```python
from build123d import *

# Parameters (mm, degrees)
SKETCH2_R           = 88.9
BOSS_EXTRUDE1_DEPTH = 3.175
SKETCH3_R           = 3.175
SKETCH3_W           = 50.8
SKETCH3_H           = 71.12
CUT_EXTRUDE1_DEPTH  = 3.175
FILLET1_R           = 22.86
SKETCH6_R           = 6.35
CUT_EXTRUDE3_DEPTH  = 126.763669734
SKETCH8_R           = 3.175
CUT_EXTRUDE4_DEPTH  = 10


with BuildPart() as part:
    # Sketch2 → Boss-Extrude1 (new body)
    with BuildSketch(Plane(origin=(0, 0, 0), x_dir=(1, 0, 0), z_dir=(0, 1, 0))):
        with Locations(Location((0, 0, 0), (0, 0, 270))):
            Circle(SKETCH2_R)
    extrude(amount=BOSS_EXTRUDE1_DEPTH)

    # Sketch3 → Cut-Extrude1 (cut)
    with BuildSketch(Plane(origin=(0, 3.175, 0), x_dir=(1, 0, 0), z_dir=(0, 1, 0))):
        with Locations(Location((65.549718535, -24.13, 0), (0, 0, 270))):
            Circle(SKETCH3_R)
        with Locations(Location((65.549718535, 24.13, 0), (0, 0, 270))):
            Circle(SKETCH3_R)
        with Locations(Location((-53.672052261, 44.702721462, 0), (0, 0, 270))):
            Circle(SKETCH3_R)
        with Locations(Location((-11.877666274, 68.832721462, 0), (0, 0, 270))):
            Circle(SKETCH3_R)
        with Locations(Location((-11.877666274, -68.832721462, 0), (0, 0, 270))):
            Circle(SKETCH3_R)
        with Locations(Location((-53.672052261, -44.702721462, 0), (0, 0, 270))):
            Circle(SKETCH3_R)
        with Locations((-63.5, 0)):
            Rectangle(SKETCH3_W, SKETCH3_H)
    extrude(amount=-CUT_EXTRUDE1_DEPTH, mode=Mode.SUBTRACT)

    # Fillet1
    fillet1_edges = [part.edges().sort_by_distance(p)[0] for p in [
        (-38.1, 1.5875, 35.56),
        (-38.1, 1.5875, -35.56),
    ]]
    fillet(fillet1_edges, radius=FILLET1_R)

    # Sketch6 → Cut-Extrude3 (cut, through all)
    with BuildSketch(Plane(origin=(0, 3.175, 0), x_dir=(1, 0, 0), z_dir=(0, 1, 0))):
        with Locations(Location((65.549718535, 0, 0), (0, 0, 270))):
            Circle(SKETCH6_R)
        with BuildLine():
            Line((8.442333726, 75.182721462), (33.842333726, 75.182721462))
            ThreePointArc((33.842333726, 75.182721462), (40.192333726, 68.832721462), (33.842333726, 62.482721462))
            Line((33.842333726, 62.482721462), (8.442333726, 62.482721462))
            ThreePointArc((8.442333726, 62.482721462), (2.092333726, 68.832721462), (8.442333726, 75.182721462))
        make_face()
        with BuildLine():
            Line((8.442333726, -62.482721462), (33.842333726, -62.482721462))
            ThreePointArc((33.842333726, -62.482721462), (40.192333726, -68.832721462), (33.842333726, -75.182721462))
            Line((33.842333726, -75.182721462), (8.442333726, -75.182721462))
            ThreePointArc((8.442333726, -75.182721462), (2.092333726, -68.832721462), (8.442333726, -62.482721462))
        make_face()
    extrude(amount=-CUT_EXTRUDE3_DEPTH, mode=Mode.SUBTRACT)

    # Sketch8 → Cut-Extrude4 (cut)
    with BuildSketch(Plane(origin=(0, 3.175, 0), x_dir=(1, 0, 0), z_dir=(0, 1, 0))):
        with Locations(Location((59.175, 42, 0), (0, 0, 270))):
            Circle(SKETCH8_R)
    cut_extrude4 = extrude(amount=-CUT_EXTRUDE4_DEPTH, mode=Mode.SUBTRACT)

    # Mirror1: Cut-Extrude4 across plane
    add(cut_extrude4.mirror(Plane.XY), mode=Mode.SUBTRACT)


solid = part.part
```
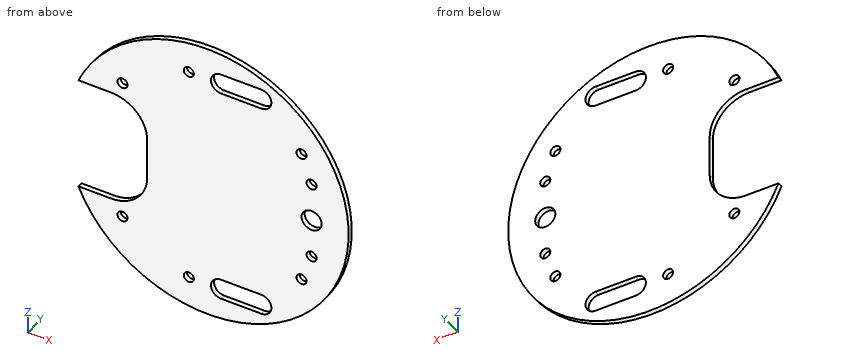
Work out the finished part from the listing and answer in its coordinate system (mm). Give positions to 0.01 mm unless a question says otherwise; leave off trailing zeros. Loops run counter-clockwise (first coordinate to the right, second up) from the corner with the lowest first, then second, coordinate; pieces in that order, holes last. Notation, with made-up numbers: (26.5, -33.5) -> (45.5, -33.5) arc R17 ccw to (45.5, -7.5) -> close; hole circle Ø11 at (39.5, 69.5). An arc over 180 degrees is marked (long way). Put each result on its own line as item: value. Start each with the question number.
Item 1: Find the intervals of material crossed by L1, parallel to Z at x = 63, y = 0.75; L2, parallel to Z at x = 18, y = 0.45; L3, parallel to X at y = 1.6, z = -42, in increasing order. Write a range as [from, to].
Item 2: The part is cut by section B-B (x = -65.5). Give the vertices of the cut face in (y, z) (3 decimals), then the cut area to 3 significant figures.
Item 3: Each of these flat-tipped pins is pushed along its axis until it touches: P1, Ø1, axis at x = 19.5, y = 2, coming from the +Z side; P2, Ø1, axis at x = -56.5, y = 0.5, coming from the +Z side (3 decimals); P3, Ø1.6, axis at x = 23, y = 2, coming from the -Z side. Where does it stop, or does it pass through?
Item 4: The part is cut by section D-D (z = 58.5). Give the vertices of the cut face in (x, y) (3 decimals).
Item 5: The part is cut by section C-C (y = 1.9). State how many separate pieces and enclosed holes the cut face has, then the cut area to 3 significant figures.
Item 6: The part is cut by section A-A (z = 24.13). Give the vertices of the cut face in (x, y) (3 decimals).
Answers below:
1. L1: [-62.72, -26.02], [-22.24, -5.82], [5.82, 22.24], [26.02, 62.72]
1. L2: [-87.06, -75.18], [-62.48, 62.48], [75.18, 87.06]
1. L3: [-78.35, -55.34], [-52.01, 56], [62.35, 78.35]
2. outline: (0, -60.108) -> (3.175, -60.108) -> (3.175, -35.56) -> (0, -35.56) -> close; (0, 35.56) -> (3.175, 35.56) -> (3.175, 60.108) -> (0, 60.108) -> close
2. area: 156 mm2
3. P1: z = 86.85
3. P2: z = 69.045
3. P3: z = -86.08
4. outline: (-66.94, 0) -> (66.94, 0) -> (66.94, 3.175) -> (-66.94, 3.175) -> close
5. separate pieces: 1
5. enclosed holes: 11
5. area: 20,300 mm2
6. outline: (-41.163, 0) -> (62.375, 0) -> (62.375, 3.175) -> (-41.163, 3.175) -> close; (68.725, 0) -> (85.563, 0) -> (85.563, 3.175) -> (68.725, 3.175) -> close
